```python
from build123d import *

# Parameters (mm, degrees)
PAD_DEPTH     = 2
SKETCH001_R   = 9.3
SKETCH001_R_2 = 9.1
PAD001_DEPTH  = 8


with BuildPart() as part:
    # Sketch → Pad (new body)
    with BuildSketch(Plane.XZ):
        Polygon((10, 0), (10, -10), (0, -10), (0, -6.5), (3.5, -6.5), (3.5, -8), (6.5, -8), (6.5, -2), (3.5, -2), (3.5, -3.5), (0, -3.5), (0, 0), (0, 38), (38, 38), (38, 0.5), (38, -3.005), (41.505, -3.005), (41.505, -1.505), (44.405, -1.505), (44.405, -7.995), (41.505, -7.995), (41.505, -6.495), (38, -6.495), (38, -10), (34, -10), (34, 0), align=None)
    extrude(amount=PAD_DEPTH)

    # Sketch001 (on Face28 of Pad) → Pad001 (join)
    with BuildSketch(Plane.XZ.offset(2)):
        with Locations((9.5, 9.5)):
            Circle(SKETCH001_R)
        with Locations((9.5, 9.5)):
            Circle(SKETCH001_R_2, mode=Mode.SUBTRACT)
    extrude(amount=PAD001_DEPTH)


solid = part.part
```
Check sheet for the modelled part. Datum: model origin and axes. Units: mm. A direction names the side the tool comes from. Round coordinates to 2 decimals unless told otherwise and drop trailing zeros. Loops run counter-clockwise (first coordinate to the right, second up) from the corner with the lowest first, then second, coordinate; pieces in that order, holes last. Notation, with made-up numbers: (-12.5, 5.25) -> (46.5, 5.25) arc R33 cw to (46.5, 39.25) -> close; hole circle Ø4 at (39, 43.25). An arc over 180 degrees is marked (long way). Write item = value, one per line. Start each with the question number.
1) Gauge pin test, flat ends, axial feed: pin 1 Ø5.5 at (x, z) = (10.5, 11.5) entering from -Y; pin 2 Ø6 at (x, y) = (18, -6.5) entering from -Z; pin 3 Ø3 at (y, z) = (-4.5, 7) entering from +X; pin 4 Ø5 at (x, y) = (32, -6.5) entering from +Z. Record the tip position at first contact, or that the pin passes through.
2) Sectioned sample at C-C, the plane x = 28. Record the cut outline in (y, z), plus the area to 3 significant figures.
3) Release check for a two-part mould opening along Z. For faces 1 (the flat face through (3.5, -1, -7)), 2 (the cylindrical face through (18.37, -5.94, 12.29)), 3 (the flat face through (38, -1, 17)), 4 (the flat face through (40, -1, -6.495)) record: released by +Z, released by -Z, zero draft, split by the parting line, or undercut.
4) Sectioned sample at A-A, the plane z = 9.5. Record the cut outline in (x, y).
5) Sectioned sample at B-B, the plane y = -7.75. Record the cut outline in (x, z).
6) Thickness scan on probe 1 along Z at (x, y) = (9.5, -4); probe 2 along Y at (x, z) = (10.5, 34); probe 3 along Z at (x, y) = (11, -4.25). Record the ranges inside material, lowest first.
7) Sectioned sample at D-D, the plane z = 24.5. Record the cut outline in (x, y).
8) Set-up check for faces 5 (the flat face through (5, -1, -2)), 6 (the flat face through (43, -1, -7.995)), 7 (the flat face through (2, -1, -3.5)), 8 (the flat face through (10, -2, 10)), 9 (the flat face through (10, -1, -5)): record each of +Z, -Z, +X, -X, +Y, -Y from which the full face is reachable in a straight line by a thin tool's end or side.
Results are:
q1.pin_1 = -2
q1.pin_2 = 2
q1.pin_3 = 18.75
q1.pin_4 = through
q2.outline = (-2, 0) -> (0, 0) -> (0, 38) -> (-2, 38) -> close
q2.area = 76.0 mm^2
q3.face_1 = undercut
q3.face_2 = split by the parting line
q3.face_3 = zero draft
q3.face_4 = released by -Z
q4.outline = (0, -2) -> (0.2, -2) -> (0.2, -10) -> (0.4, -10) -> (0.4, -2) -> (18.6, -2) -> (18.6, -10) -> (18.8, -10) -> (18.8, -2) -> (38, -2) -> (38, 0) -> (0, 0) -> close
q5.outline = circle Ø18.6 at (9.5, 9.5); hole circle Ø18.2 at (9.5, 9.5)
q6.probe_1 = 0.2 to 0.4, 18.6 to 18.8
q6.probe_2 = -2 to 0
q6.probe_3 = 0.32 to 0.52, 18.48 to 18.68
q7.outline = (0, -2) -> (38, -2) -> (38, 0) -> (0, 0) -> close
q8.face_5 = +Y, -Y
q8.face_6 = -Z, +X, +Y, -Y
q8.face_7 = -X, +Y, -Y
q8.face_8 = -Y
q8.face_9 = -Z, +Y, -Y
